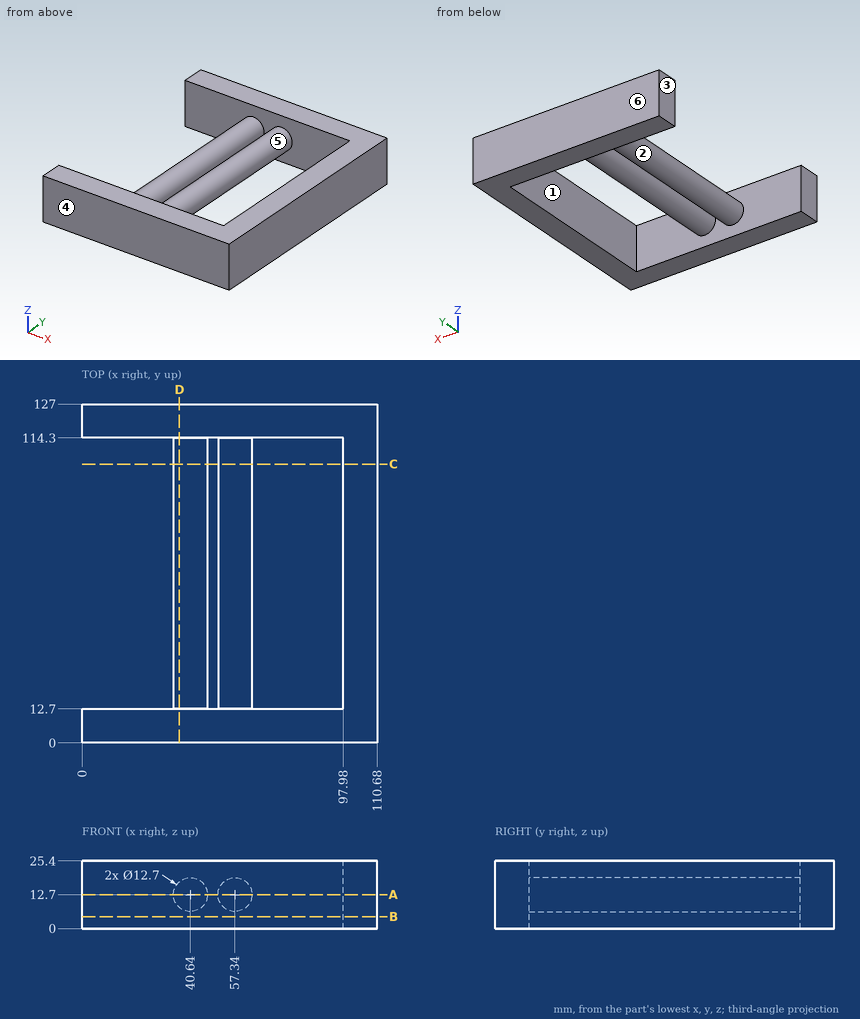
Print and shaded views of the part. All mm, measured from the part's lowest x, y and z. A direction names the side the tool comes from. Round coordinates to 2 decimals unless told otherwise and drop trailing zeros. Write each loop counter-clockwise with the first axis right and the second up, starting at its lowest first coordinate (ties: lowest second). Pieces come first, ordered by that corner, then holes.
Item 1: Two-plate mould, pull along X, no slides. Class the marked faces 1, 2, 3 and 4: +X half, -X half, draft (parallel to the pull), parting line (faces both ways), or undercut.
Results:
face 1: undercut
face 2: undercut
face 3: -X half
face 4: draft
Item 2: Which spindle directions (+Z, -Z, +X, -X, +Y, -Y) get a long thin tool onto all of the face, cutting with end or side? Do the marked faces 5 and 6. Say none if no direction does.
Results:
face 5: none
face 6: +Z, -Z, +X, -X, +Y
Item 3: Cut at C-C, the plane y = 104.5. Give the cut face in (x, z), plus the area to 3 significant figures.
Results:
outline: circle Ø12.7 at (40.64, 12.7); circle Ø12.7 at (57.34, 12.7); (97.98, 0) - (110.68, 0) - (110.68, 25.4) - (97.98, 25.4) - close
area: 576 mm2
Item 4: Drop flat-ended pins along their axis: pin 1 Ø5 at (y, z) = (98, 17.5) entering from -X; pin 2 Ø1 at (x, y) = (64.5, 81) entering from +Z; pin 3 Ø4 at (y, z) = (112, 9.5) entering from -X. Give the stop position or say it passes through.
Results:
pin 1: stops at x = 34.72
pin 2: passes through
pin 3: stops at x = 34.4
Item 5: Cut at D-D, the plane x = 36.5. Give the cut face in (y, z).
Results:
outline: (0, 0) - (12.7, 0) - (12.7, 7.89) - (114.3, 7.89) - (114.3, 0) - (127, 0) - (127, 25.4) - (114.3, 25.4) - (114.3, 17.51) - (12.7, 17.51) - (12.7, 25.4) - (0, 25.4) - close
Item 6: Probe L1, parallel to X at y = 26.5, z = 13; L2, parallel to Y at x = 58, z = 23.75; L3, parallel to X at y = 63.5, z = 11.75. List the from-to ranges inside material, lowest first.
Results:
L1: x = 34.3 to 46.98, 51 to 63.68, 97.98 to 110.68
L2: y = 0 to 12.7, 114.3 to 127
L3: x = 34.36 to 46.92, 51.06 to 63.62, 97.98 to 110.68
Item 7: Cut at B-B, the plane z = 4.5. Give the cut face in (x, y), plus the area to 3 significant figures.
Results:
outline: (0, 0) - (110.68, 0) - (110.68, 127) - (0, 127) - (0, 114.3) - (97.98, 114.3) - (97.98, 12.7) - (0, 12.7) - close
area: 4,100 mm2
Item 8: Cut at A-A, the plane z = 12.7. Give the cut face in (x, y).
Results:
outline: (0, 0) - (110.68, 0) - (110.68, 127) - (0, 127) - (0, 114.3) - (34.29, 114.3) - (34.29, 12.7) - (0, 12.7) - close; hole (46.99, 12.7) - (50.99, 12.7) - (50.99, 114.3) - (46.99, 114.3) - close; hole (63.69, 12.7) - (97.98, 12.7) - (97.98, 114.3) - (63.69, 114.3) - close
